Here's how the part is built. I have some questions about the finished solid (model axes, mm). Face numbers are marked on the shaded views. A direction names the side the tool comes from. Give positions to 0.01 mm unless a question says otherwise; leave off trailing zeros. Order: outer loops, then holes, each group sorted by start corner. A loop starts at its lowest first (then second) coordinate and runs counter-clockwise, first axis right, second up. Notation, with made-up numbers: M -35,-34 L -30,-34 A22 cw -30,-22 Z; hole C 21,-34 d11. An arc over 180 degrees is marked long. One line per item, written item: value. Start each with the question number.
from build123d import *

# Parameters (mm, degrees)
F0_R     = 2.5
F0_R_2   = 1.25
F1_DEPTH = 10
F3_DEPTH = 3


with BuildPart() as f1:
    # F0 (on Top) → F1 (new body)
    with BuildSketch(Plane.XY):
        Circle(F0_R)
        Circle(F0_R_2, mode=Mode.SUBTRACT)
    extrude(amount=F1_DEPTH)

    # F2 (on face) → F3 (cut)
    with BuildSketch(Plane.XY.offset(10)):
        with BuildLine():
            Line((-1.1456439237, 0.5), (-2.4494897428, 0.5))
            ThreePointArc((-2.4494897428, 0.5), (-2.5, 0), (-2.4494897428, -0.5))
            Line((-2.4494897428, -0.5), (-1.1456439237, -0.5))
            ThreePointArc((-1.1456439237, -0.5), (-1.25, 0), (-1.1456439237, 0.5))
        make_face()
        with BuildLine():
            ThreePointArc((2.5, 0), (2.4873403825, 0.251272405), (2.4494897428, 0.5))
            Line((2.4494897428, 0.5), (1.1456439237, 0.5))
            ThreePointArc((1.1456439237, 0.5), (1.2236328912, 0.2553870546), (1.25, 0))
            ThreePointArc((1.25, 0), (1.2236328912, -0.2553870546), (1.1456439237, -0.5))
            Line((1.1456439237, -0.5), (2.4494897428, -0.5))
            ThreePointArc((2.4494897428, -0.5), (2.4873403825, -0.251272405), (2.5, 0))
        make_face()
    extrude(amount=-F3_DEPTH, mode=Mode.SUBTRACT)


solid = f1.part
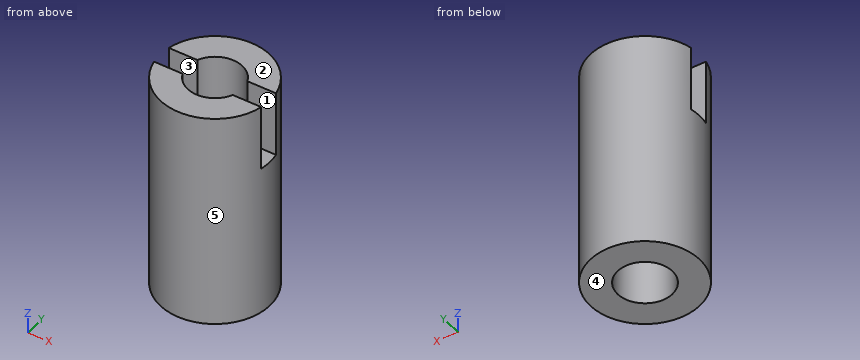
Item 1: We'd pull the mould along Y, two halves only. Please class the marked faces 3, 4 and 5: +Y half, -Y half, draft (parallel to the pull), parting line (faces both ways), or undercut.
Item 2: Will these pins go through, and if not, where does the flat tip stop? P1, Ø1.5, axis at x = -2, z = 2.5, coming from the +Y side; P2, Ø1.5, axis at y = 1, z = 5, coming from the +X side; P3, Ø0.5, axis at x = -2, y = 0, coming from the +Z side.
Item 3: I want a section at B-B on y = 0. Write out the boundary of the cut face in (x, z).
Item 4: I want a section at D-D on z = 1.5. Write out the boundary of the cut face in (x, y).
Item 5: I want a section at C-C on x = 2. Write out the boundary of the cut face in (y, z), plus the area to 3 significant figures.
Item 6: Please list where these lines run through material, in increasing order: probe 1 along Y at (x, z) = (0, 6.5); probe 2 along X at (y, z) = (-0.25, 6.25); probe 3 along X at (y, z) = (-0.65, 1.75). Write a range as [from, to].
Item 7: For the marked faces 1 and 2, which set-ups out of +Z, -Z, +X, -X, +Y, -Y let a thin tool reach every point of the face, with its end or its side?
Item 8: I want a section at A-A on z = 9. Write out the boundary of the cut face in (x, y).
Answer below:
1. face 3: undercut
1. face 4: draft
1. face 5: parting line
2. P1: stops at y = 2.17
2. P2: stops at x = 2.49
2. P3: stops at z = 7
3. outline: M -2.5,0 L -1.25,0 L -1.25,7 L -2.5,7 Z; M 1.25,0 L 2.5,0 L 2.5,7 L 1.25,7 Z
4. outline: C 0,0 d5; hole C 0,0 d2.5
5. outline: M -1.5,0 L 1.5,0 L 1.5,10 L 0.5,10 L 0.5,7 L -0.5,7 L -0.5,10 L -1.5,10 Z
5. area: 27.0 mm²
6. probe 1: y = [-2.5, -1.25], [1.25, 2.5]
6. probe 2: x = [-2.49, -1.22], [1.22, 2.49]
6. probe 3: x = [-2.41, -1.07], [1.07, 2.41]
7. face 1: +Z, +X, -X
7. face 2: +Z, +X, -X, +Y, -Y
8. outline: M -2.45,-0.5 A2.5 ccw 2.45,-0.5 L 1.15,-0.5 A1.25 cw -1.15,-0.5 Z; M -2.45,0.5 L -1.15,0.5 A1.25 cw 1.15,0.5 L 2.45,0.5 A2.5 ccw Z
